```python
from build123d import *

# Parameters (mm, degrees)
SKIZZE1_W                                 = 110
SKIZZE1_H                                 = 170
AUFSATZ_LINEAR_AUSTRAGEN1_DEPTH           = 5
VERRUNDUNG1_R                             = 5
SKIZZE7_W                                 = 12
SKIZZE7_H                                 = 16
AUFSATZ_LINEAR_AUSTRAGEN3_DEPTH           = 21
VERRUNDUNG2_R                             = 2
SKIZZE8_R                                 = 4.2
SCHNITT_LINEAR_AUSTRAGEN3_DEPTH           = 105.527508341
LINEARES_MUSTER1_COUNT                    = 2
LINEARES_MUSTER1_PITCH                    = 134
LINEARES_MUSTER1_COUNT_DIR2               = 2
LINEARES_MUSTER1_PITCH_DIR2               = 98
SKIZZE11_W                                = 78
SKIZZE11_H                                = 150
SKIZZE11_W_2                              = 75
SKIZZE11_H_2                              = 147
AUFSATZ_LINEAR_AUSTRAGEN4_DEPTH           = 2
VERRUNDUNG3_R                             = 1
SKIZZE12_W                                = 8
SKIZZE12_H                                = 25
SCHNITT_LINEAR_AUSTRAGEN4_DEPTH           = 104.397292034
SKIZZE13_R                                = 1.75
AUFSATZ_LINEAR_AUSTRAGEN5_DEPTH           = 4
AUFSATZ_LINEAR_AUSTRAGEN5_DRAFT           = 2
AUFSATZ_LINEAR_AUSTRAGEN5_PROFILE_2_DEPTH = 4
AUFSATZ_LINEAR_AUSTRAGEN5_PROFILE_2_DRAFT = 2
AUFSATZ_LINEAR_AUSTRAGEN5_PROFILE_3_DEPTH = 4
AUFSATZ_LINEAR_AUSTRAGEN5_PROFILE_3_DRAFT = 2
AUFSATZ_LINEAR_AUSTRAGEN5_PROFILE_4_DEPTH = 4
AUFSATZ_LINEAR_AUSTRAGEN5_PROFILE_4_DRAFT = 2
SKIZZE14_R                                = 2
SCHNITT_LINEAR_AUSTRAGEN5_DEPTH           = 4.5
VERRUNDUNG4_R                             = 1


with BuildPart() as part:
    # Skizze1 → Aufsatz-Linear austragen1 (new body)
    with BuildSketch(Plane.XY):
        Rectangle(SKIZZE1_W, SKIZZE1_H)
    extrude(amount=AUFSATZ_LINEAR_AUSTRAGEN1_DEPTH)

    # Verrundung1
    verrundung1_edges = [part.edges().sort_by_distance(p)[0] for p in [
        (55, -85, 2.5),
        (-55, -85, 2.5),
        (-55, 85, 2.5),
        (55, 85, 2.5),
    ]]
    fillet(verrundung1_edges, radius=VERRUNDUNG1_R)

    # Skizze7 → Aufsatz-Linear austragen3 (add)
    with BuildSketch(Plane.XY.offset(5)):
        with Locations((-49, 65)):
            Rectangle(SKIZZE7_W, SKIZZE7_H)
        with Locations((49, 65)):
            Rectangle(SKIZZE7_W, SKIZZE7_H)
        with Locations((49, -65)):
            Rectangle(SKIZZE7_W, SKIZZE7_H)
        with Locations((-49, -65)):
            Rectangle(SKIZZE7_W, SKIZZE7_H)
    extrude(amount=AUFSATZ_LINEAR_AUSTRAGEN3_DEPTH)

    # Verrundung2
    verrundung2_edges = [part.edges().sort_by_distance(p)[0] for p in [
        (-49, 57, 5),
        (-43, 65, 5),
        (-49, 73, 5),
        (49, 73, 5),
        (43, 65, 5),
        (49, 57, 5),
        (49, -57, 5),
        (43, -65, 5),
        (49, -73, 5),
        (-49, -73, 5),
        (-43, -65, 5),
        (-49, -57, 5),
    ]]
    fillet(verrundung2_edges, radius=VERRUNDUNG2_R)

    # Skizze8 → Schnitt-Linear austragen3 (cut, through all)
    with BuildSketch(Plane.XY.offset(26)):
        with Locations((-49, 67)):
            Circle(SKIZZE8_R)
    schnitt_linear_austragen3 = extrude(amount=-SCHNITT_LINEAR_AUSTRAGEN3_DEPTH, mode=Mode.SUBTRACT)

    # Lineares Muster1: Schnitt-Linear austragen3 2 × 2
    with Locations(*[(j * LINEARES_MUSTER1_PITCH_DIR2, -i * LINEARES_MUSTER1_PITCH, 0) for i in range(LINEARES_MUSTER1_COUNT) for j in range(LINEARES_MUSTER1_COUNT_DIR2) if (i, j) != (0, 0)]):
        add(schnitt_linear_austragen3, mode=Mode.SUBTRACT)

    # Skizze11 → Aufsatz-Linear austragen4 (add)
    with BuildSketch(Plane.XY.offset(5)):
        with Locations((0, -6.5)):
            Rectangle(SKIZZE11_W, SKIZZE11_H)
        with Locations((0, -6.5)):
            Rectangle(SKIZZE11_W_2, SKIZZE11_H_2, mode=Mode.SUBTRACT)
    extrude(amount=AUFSATZ_LINEAR_AUSTRAGEN4_DEPTH)

    # Verrundung3
    verrundung3_edges = [part.edges().sort_by_distance(p)[0] for p in [
        (39, -81.5, 6),
        (39, 68.5, 6),
        (-39, 68.5, 6),
        (-39, -81.5, 6),
        (37.5, 67, 6),
        (-37.5, 67, 6),
        (-37.5, -80, 6),
        (37.5, -80, 6),
    ]]
    fillet(verrundung3_edges, radius=VERRUNDUNG3_R)

    # Skizze12 → Schnitt-Linear austragen4 (cut, through all)
    with BuildSketch(Plane.XY.offset(5)):
        with Locations((-44, 37.5)):
            Rectangle(SKIZZE12_W, SKIZZE12_H)
        with Locations((44, 37.5)):
            Rectangle(SKIZZE12_W, SKIZZE12_H)
        with Locations((44, -37.5)):
            Rectangle(SKIZZE12_W, SKIZZE12_H)
        with Locations((-44, -37.5)):
            Rectangle(SKIZZE12_W, SKIZZE12_H)
    extrude(amount=-SCHNITT_LINEAR_AUSTRAGEN4_DEPTH, mode=Mode.SUBTRACT)


with BuildPart() as aufsatz_linear_austragen5_tool:
    # Skizze13 → Aufsatz-Linear austragen5 (with draft: the straight prism first)
    with BuildSketch(Plane.XY.offset(26)):
        with Locations((-49, 59.5)):
            Circle(SKIZZE13_R)
    extrude(amount=AUFSATZ_LINEAR_AUSTRAGEN5_DEPTH)
    # Aufsatz-Linear austragen5: the draft: its side faces are tilted about the plane it starts from
    aufsatz_linear_austragen5_sides = [aufsatz_linear_austragen5_tool.faces().sort_by_distance(p)[0] for p in [
        (-50.75, 59.5, 28),
    ]]
    draft(aufsatz_linear_austragen5_sides, Plane.XY.offset(26), AUFSATZ_LINEAR_AUSTRAGEN5_DRAFT)


with BuildPart() as part_1:
    add(part.part)

    # Aufsatz-Linear austragen5: add aufsatz_linear_austragen5_tool
    add(aufsatz_linear_austragen5_tool.part)


with BuildPart() as aufsatz_linear_austragen5_profile_2_tool:
    # Skizze13 → Aufsatz-Linear austragen5 profile 2 (with draft: the straight prism first)
    with BuildSketch(Plane.XY.offset(26)):
        with Locations((49, 59.5)):
            Circle(SKIZZE13_R)
    extrude(amount=AUFSATZ_LINEAR_AUSTRAGEN5_PROFILE_2_DEPTH)
    # Aufsatz-Linear austragen5 profile 2: the draft: its side faces are tilted about the plane it starts from
    aufsatz_linear_austragen5_profile_2_sides = [aufsatz_linear_austragen5_profile_2_tool.faces().sort_by_distance(p)[0] for p in [
        (47.25, 59.5, 28),
    ]]
    draft(aufsatz_linear_austragen5_profile_2_sides, Plane.XY.offset(26), AUFSATZ_LINEAR_AUSTRAGEN5_PROFILE_2_DRAFT)


with BuildPart() as part_2:
    add(part_1.part)

    # Aufsatz-Linear austragen5 profile 2: add aufsatz_linear_austragen5_profile_2_tool
    add(aufsatz_linear_austragen5_profile_2_tool.part)


with BuildPart() as aufsatz_linear_austragen5_profile_3_tool:
    # Skizze13 → Aufsatz-Linear austragen5 profile 3 (with draft: the straight prism first)
    with BuildSketch(Plane.XY.offset(26)):
        with Locations((49, -59.5)):
            Circle(SKIZZE13_R)
    extrude(amount=AUFSATZ_LINEAR_AUSTRAGEN5_PROFILE_3_DEPTH)
    # Aufsatz-Linear austragen5 profile 3: the draft: its side faces are tilted about the plane it starts from
    aufsatz_linear_austragen5_profile_3_sides = [aufsatz_linear_austragen5_profile_3_tool.faces().sort_by_distance(p)[0] for p in [
        (47.25, -59.5, 28),
    ]]
    draft(aufsatz_linear_austragen5_profile_3_sides, Plane.XY.offset(26), AUFSATZ_LINEAR_AUSTRAGEN5_PROFILE_3_DRAFT)


with BuildPart() as part_3:
    add(part_2.part)

    # Aufsatz-Linear austragen5 profile 3: add aufsatz_linear_austragen5_profile_3_tool
    add(aufsatz_linear_austragen5_profile_3_tool.part)


with BuildPart() as aufsatz_linear_austragen5_profile_4_tool:
    # Skizze13 → Aufsatz-Linear austragen5 profile 4 (with draft: the straight prism first)
    with BuildSketch(Plane.XY.offset(26)):
        with Locations((-49, -59.5)):
            Circle(SKIZZE13_R)
    extrude(amount=AUFSATZ_LINEAR_AUSTRAGEN5_PROFILE_4_DEPTH)
    # Aufsatz-Linear austragen5 profile 4: the draft: its side faces are tilted about the plane it starts from
    aufsatz_linear_austragen5_profile_4_sides = [aufsatz_linear_austragen5_profile_4_tool.faces().sort_by_distance(p)[0] for p in [
        (-50.75, -59.5, 28),
    ]]
    draft(aufsatz_linear_austragen5_profile_4_sides, Plane.XY.offset(26), AUFSATZ_LINEAR_AUSTRAGEN5_PROFILE_4_DRAFT)


with BuildPart() as part_4:
    add(part_3.part)

    # Aufsatz-Linear austragen5 profile 4: add aufsatz_linear_austragen5_profile_4_tool
    add(aufsatz_linear_austragen5_profile_4_tool.part)

    # Skizze14 → Schnitt-Linear austragen5 (cut)
    with BuildSketch(Plane(origin=(0, 0, 0), x_dir=(-1, 0, 0), z_dir=(0, 0, -1))):
        with Locations((49, 59.5)):
            Circle(SKIZZE14_R)
        with Locations(Location((-49, 59.5, 0), (0, 0, 180))):
            Circle(SKIZZE14_R)
        with Locations((-49, -59.5)):
            Circle(SKIZZE14_R)
        with Locations(Location((49, -59.5, 0), (0, 0, 180))):
            Circle(SKIZZE14_R)
    extrude(amount=-SCHNITT_LINEAR_AUSTRAGEN5_DEPTH, mode=Mode.SUBTRACT)

    # Verrundung4
    verrundung4_edges = [part_4.edges().sort_by_distance(p)[0] for p in [
        (-48, -50, 2.5),
        (-48, -25, 2.5),
        (-40, -25, 2.5),
        (-40, -50, 2.5),
        (40, -25, 2.5),
        (48, -25, 2.5),
        (48, -50, 2.5),
        (40, -50, 2.5),
        (48, 50, 2.5),
        (48, 25, 2.5),
        (40, 25, 2.5),
        (40, 50, 2.5),
        (-40, 50, 2.5),
        (-40, 25, 2.5),
        (-48, 25, 2.5),
        (-48, 50, 2.5),
    ]]
    fillet(verrundung4_edges, radius=VERRUNDUNG4_R)


solid = part_4.part
```
For this review, take the finished solid that the model builds, in its own axes (mm). A direction names the side the tool comes from. Round coordinates to 2 decimals unless told otherwise and drop trailing zeros. Write each loop counter-clockwise with the first axis right and the second up, starting at its lowest first coordinate (ties: lowest second). Pieces come first, ordered by that corner, then holes. Notation, with made-up numbers: (45, -0.5) - (86, -0.5) arc R32 ccw to (86, 33.5) - close; hole circle Ø1 at (83.5, -1). An arc over 180 degrees is marked (long way). Answer as CSV lines item,"result". Start each with the question number.
(1) Add section C-C, the plane x = 9.5. State the section outline as (y, z) points.
(2) Machinability: for faces 1 (the flat face through (-49, -57, 16)), 2 (the flat face through (-40, 37, 3)), 3 (the cylindrical face through (48.74, 57.517, 2.218)), 4 (the flat face through (49, 73, 16)), 5 (the conical face through (-50.239, 60.636, 27.972)), which of the approach directions +Z, -Z, +X, -X, +Y, -Y give a long, thin tool a straight path to every point of the face, cutting with its end or side? Answer none if there is none.
(3) Mouldability with a two-part tool opening along X and no side actions: class faces 6 (the cylindrical face through (54, 83, 3)), 7 (the flat face through (-52, 63, 26)), 8 (the flat face through (-49, -59, 30)) as +X half, -X half, draft (parallel to the pull), parting line (faces both ways), or undercut.
(4) For pin 1 (8 mm diameter, centred on y = 29, z = 7.5, fed in from +X); pin 2 (1.6 mm diameter, centred on y = 29.5, z = 6.5, fed in from -X); pin 3 (1 mm diameter, centred on x = -31, z = 6.5, fed in from -Y); pin 4 (13 mm diameter, centred on x = -46, z = 17, fed in from +Y), all flat-tipped, find the tip position at first contact; note any pin that passes through.
(5) Add section D-D, the plane y = -15.5. State the section outline as (x, z) points.
(6) For line 1 (Y direction, x = -49, z = 18.5); line 2 (Y direction, x = 49, z = 3.1); line 3 (X direction, y = -24, z = 6.5), list the stretches that pass through material, from the lowest coordinate up.
(7) Add section A-A, the plane y = 42. State the section outline as (x, z) points.
(8) Add section B-B, the plane z = 16.5. State the section outline as (x, y) points, plus the area to 3 significant figures.
From the geometry:
1,outline,"(-85, 0) - (85, 0) - (85, 5) - (68.5, 5) - (68.5, 7) - (67, 7) - (67, 5) - (-80, 5) - (-80, 7) - (-81.5, 7) - (-81.5, 5) - (-85, 5) - close"
2,face 1,"+Z, +X, -X"
2,face 2,"+Z, -Z"
2,face 3,"-Z"
2,face 4,"+Z, +X, -X, +Y"
2,face 5,"+Z"
3,face 6,"+X half"
3,face 7,"undercut"
3,face 8,"draft"
4,pin 1,"stops at x = 55"
4,pin 2,"stops at x = -39"
4,pin 3,"stops at y = -81.5"
4,pin 4,"stops at y = 73"
5,outline,"(-55, 0) - (55, 0) - (55, 5) - (39, 5) - (39, 7) - (37.5, 7) - (37.5, 5) - (-37.5, 5) - (-37.5, 7) - (-39, 7) - (-39, 5) - (-55, 5) - close"
6,line 1,"y = -73 to -71.2, -62.8 to -57, 57 to 62.8, 71.2 to 73"
6,line 2,"y = -85 to -71.2, -62.8 to -61.5, -57.5 to 57.5, 61.5 to 62.8, 71.2 to 85"
6,line 3,"x = -39 to -37.5, 37.5 to 39"
7,outline,"(-55, 0) - (-48, 0) - (-48, 5) - (-55, 5) - close; (-40, 0) - (40, 0) - (40, 5) - (39, 5) - (39, 7) - (37.5, 7) - (37.5, 5) - (-37.5, 5) - (-37.5, 7) - (-39, 7) - (-39, 5) - (-40, 5) - close; (48, 0) - (55, 0) - (55, 5) - (48, 5) - close"
8,outline,"(-55, -73) - (-43, -73) - (-43, -57) - (-55, -57) - close; (-55, 57) - (-43, 57) - (-43, 73) - (-55, 73) - close; (43, -73) - (55, -73) - (55, -57) - (43, -57) - close; (43, 57) - (55, 57) - (55, 73) - (43, 73) - close; hole circle Ø8.4 at (-49, -67); hole circle Ø8.4 at (-49, 67); hole circle Ø8.4 at (49, -67); hole circle Ø8.4 at (49, 67)"
8,area,"546 mm²"
